The model under review builds one solid part; all positions refer to its coordinate system, in mm. Coordinates: 2 decimals unless noted, no trailing zeros. Order: outer loops, then holes, each group sorted by start corner. A loop starts at its lowest first (then second) coordinate and runs counter-clockwise, first axis right, second up. Notation, with made-up numbers: (-35.75, 36.25) -> (-0.75, 36.25) arc R27 cw to (-0.75, 69.25) -> close; hole circle Ø11 at (62, 71). An arc over 180 degrees is marked (long way). Use one line per item in the form item = value.
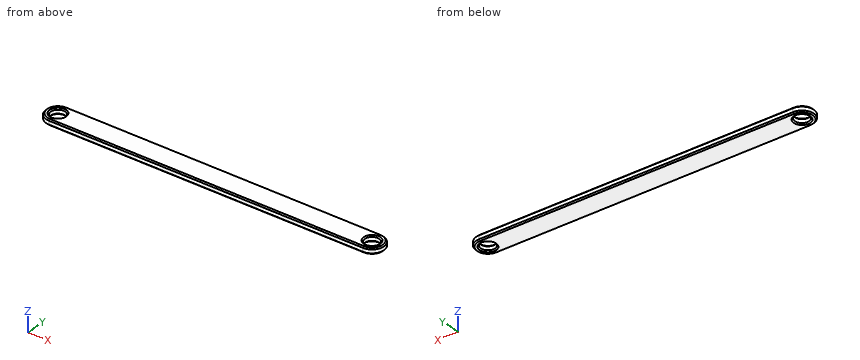
from build123d import *

# Parameters (mm, degrees)
SKETCH1_R           = 30
BOSS_EXTRUDE1_DEPTH = 25
CHAMFER1_SIZE       = 5


with BuildPart() as part:
    # Sketch1 → Boss-Extrude1 (new body)
    with BuildSketch(Plane.XY):
        with BuildLine():
            Line((662.5, -50), (-662.5, -50))
            ThreePointArc((-662.5, -50), (-712.5, 0), (-662.5, 50))
            Line((-662.5, 50), (662.5, 50))
            ThreePointArc((662.5, 50), (712.5, 0), (662.5, -50))
        make_face()
        with Locations((-662.5, 0)):
            Circle(SKETCH1_R, mode=Mode.SUBTRACT)
        with Locations(Location((662.5, 0, 0), (0, 0, 180))):
            Circle(SKETCH1_R, mode=Mode.SUBTRACT)
    extrude(amount=BOSS_EXTRUDE1_DEPTH)

    # Chamfer1
    chamfer1_edges = [part.edges().sort_by_distance(p)[0] for p in [
        (712.5, 0, 25),
        (-692.5, 0, 0),
        (-692.5, 0, 25),
        (0, 50, 25),
        (692.5, 0, 0),
        (692.5, 0, 25),
        (-712.5, 0, 25),
        (0, 50, 0),
        (712.5, 0, 0),
        (0, -50, 0),
        (-712.5, 0, 0),
        (0, -50, 25),
    ]]
    chamfer(chamfer1_edges, length=CHAMFER1_SIZE)


solid = part.part
Item 1: We need section B-B (z = 14.5). Write out the cut boundary in (x, y), plus the area to 3 significant figures.
Results found:
outline = (-662.5, -50) -> (662.5, -50) arc R50 ccw to (662.5, 50) -> (-662.5, 50) arc R50 ccw to start; hole circle Ø60 at (-662.5, 0); hole circle Ø60 at (662.5, 0)
area = 135,000 mm²
Item 2: We need section A-A (y = 0). Write out the cut boundary in (x, z), plus the area to 3 significant figures.
Results found:
outline = (-712.5, 5) -> (-707.5, 0) -> (-697.5, 0) -> (-692.5, 5) -> (-692.5, 20) -> (-697.5, 25) -> (-707.5, 25) -> (-712.5, 20) -> close; (-632.5, 5) -> (-627.5, 0) -> (627.5, 0) -> (632.5, 5) -> (632.5, 20) -> (627.5, 25) -> (-627.5, 25) -> (-632.5, 20) -> close; (692.5, 5) -> (697.5, 0) -> (707.5, 0) -> (712.5, 5) -> (712.5, 20) -> (707.5, 25) -> (697.5, 25) -> (692.5, 20) -> close
area = 32,500 mm²
Item 3: Clearance check with flat-ended pins moving along their axes: pin 1 (1.5 mm diameter, centred on y = -13, z = 16.5, fed in from +X); pin 2 (3 mm diameter, centred on y = -30.5, z = 15.5, fed in from -X); pin 3 (1 mm diameter, centred on y = 23.5, z = 21, fed in from -X). State where each tip first meets the part, or that it passes through.
Results found:
pin_1 = 710.98
pin_2 = -703.23
pin_3 = -706.13
Item 4: We need section C-C (x = -248.5). Write out the cut boundary in (y, z).
Results found:
outline = (-50, 5) -> (-45, 0) -> (45, 0) -> (50, 5) -> (50, 20) -> (45, 25) -> (-45, 25) -> (-50, 20) -> close
Item 5: To check wall thickness, follow L1, parallel to Y at x = -662.5, z = 10.5; L2, parallel to X at y = -16.5, z = 16; L3, parallel to X at y = 12.5, z = 2.25. State the ranges of each line that lie inside material, in increasing order. Write a range as from..to.
Results found:
L1 = -50..-30, 30..50
L2 = -709.7..-687.55, -637.45..637.45, 687.55..709.7
L3 = -708.07..-692.77, -632.23..632.23, 692.77..708.07
